Part print with two shaded views. Sizes in mm from the minimum x, y, z corner. A direction names the side the tool comes from. Give positions to 0.01 mm unless a question says otherwise; leave off trailing zeros. Order: outer loops, then holes, each group sorted by start corner. A loop starts at its lowest first (then second) coordinate and runs counter-clockwise, first axis right, second up. Notation, with made-up numbers: (1.5, 46.5) -> (59.5, 46.5) arc R21 cw to (59.5, 70.5) -> close; hole circle Ø7 at (44, -31.5). An arc over 180 degrees is marked (long way). Write item = value, one per line. Start each with the question number.
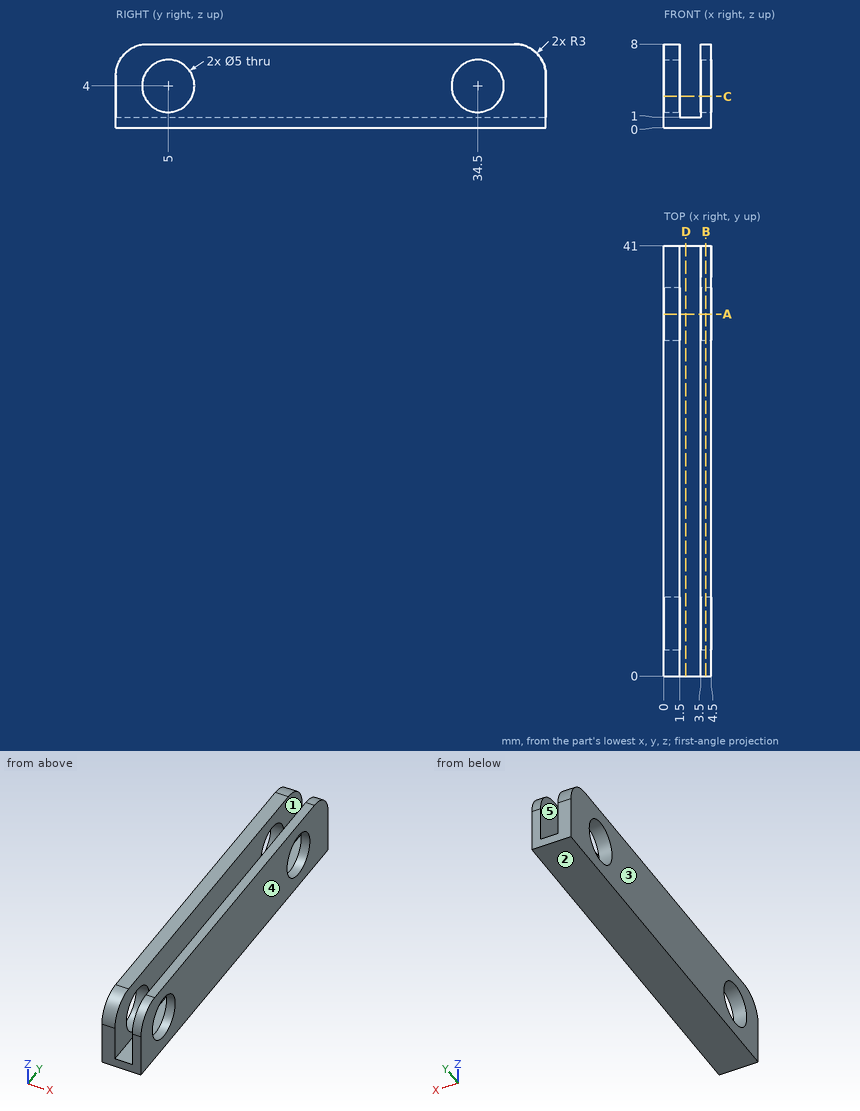
(1) Cut at B-B, the plane x = 4. Give the cut face in (y, z).
(2) Wall check: line 1 (X direction, y = 28.5, z = 2.75); line 2 (Z direction, x = 3.85, y = 34.5); line 3 (Y direction, x = 4.25, z = 5.25). Give the ranges that are in metal, low to high. Write a range as [from, to].
(3) Cut at A-A, the plane y = 34.5. Give the cut face in (x, z), plus the area to 3 significant figures.
(4) 3-axis set-ups, long thin cutter, end or side, ignore diameter. For the marked faces 1 and 2: which of +Z, -Z, +X, -X, +Y, -Y reach the whole face in a straight line?
(5) Mould opens along X. For the marked faces 3, 4 and 5 say: released by +X, released by -X, zero draft, split by the parting line, or undercut.
(6) Flat gauge pin, fed straight in: P1, Ø4, axis at y = 5, z = 4, coming from the -X side. Where does the tip first touch, or does it go through?
(7) Cut at D-D, the plane x = 2.1. Give the cut face in (y, z), plus the area to 3 significant figures.
(8) Cut at C-C, the plane z = 3. Give the cut face in (x, y), plus the area to 3 significant figures.
Results:
q1.outline = (0, 0) -> (41, 0) -> (41, 5) arc R3 ccw to (38, 8) -> (3, 8) arc R3 ccw to (0, 5) -> close; hole circle Ø5 at (5, 4); hole circle Ø5 at (34.5, 4)
q2.line_1 = [0, 1.5], [3.5, 4.5]
q2.line_2 = [0, 1.5], [6.5, 8]
q2.line_3 = [0.01, 2.83], [7.17, 32.33], [36.67, 40.99]
q3.outline = (0, 0) -> (4.5, 0) -> (4.5, 1.5) -> (3.5, 1.5) -> (3.5, 1) -> (1.5, 1) -> (1.5, 1.5) -> (0, 1.5) -> close; (0, 6.5) -> (1.5, 6.5) -> (1.5, 8) -> (0, 8) -> close; (3.5, 6.5) -> (4.5, 6.5) -> (4.5, 8) -> (3.5, 8) -> close
q3.area = 9.50 mm2
q4.face_1 = +Z, +Y, -Y
q4.face_2 = -Z, +X, -X, +Y, -Y
q5.face_3 = released by -X
q5.face_4 = released by +X
q5.face_5 = undercut
q6.P1 = through
q7.outline = (0, 0) -> (41, 0) -> (41, 1) -> (0, 1) -> close
q7.area = 41.0 mm2
q8.outline = (0, 0) -> (1.5, 0) -> (1.5, 2.71) -> (0, 2.71) -> close; (0, 7.29) -> (1.5, 7.29) -> (1.5, 32.21) -> (0, 32.21) -> close; (0, 36.79) -> (1.5, 36.79) -> (1.5, 41) -> (0, 41) -> close; (3.5, 0) -> (4.5, 0) -> (4.5, 2.71) -> (3.5, 2.71) -> close; (3.5, 7.29) -> (4.5, 7.29) -> (4.5, 32.21) -> (3.5, 32.21) -> close; (3.5, 36.79) -> (4.5, 36.79) -> (4.5, 41) -> (3.5, 41) -> close
q8.area = 79.6 mm2
